The listing builds one solid part. Answer for the finished solid, in the listing's coordinates (mm). Face numbers are marked on the shaded views. Coordinates: 2 decimals unless noted, no trailing zeros. Loops run counter-clockwise (first coordinate to the right, second up) from the corner with the lowest first, then second, coordinate; pieces in that order, holes last. Notation, with made-up numbers: (64.25, 0.5) - (122.25, 0.5) arc R20 cw to (122.25, 35.5) - close; hole circle Ø5 at (42.25, 23.25). An arc over 180 degrees is marked (long way). One line per question, with ' | ' between items.
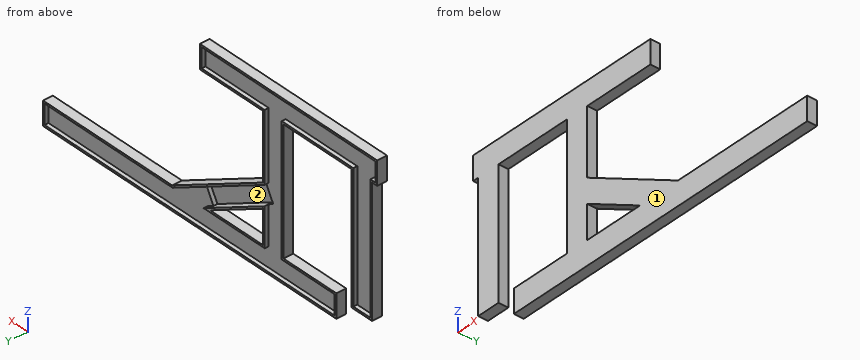
from build123d import *

# Parameters (mm, degrees)
SKETCH_3_W           = 10
SKETCH_3_H           = 65
SKETCH_3_W_2         = 85
SKETCH_3_H_2         = 10
EXTRUDE_2_DEPTH      = 1
EXTRUDE_3_DEPTH      = 4
EXTRUDE_3_DEPTH_BACK = 1
EXTRUDE_4_DEPTH      = 2
SKETCH_7_W           = 10
SKETCH_7_H           = 12
CUT_EXTRUDE_1_DEPTH  = 5
SKETCH_8_W           = 1
SKETCH_8_H           = 10
EXTRUDE_5_DEPTH      = 2
SKETCH_9_W           = 10
SKETCH_9_H           = 12
EXTRUDE_7_DEPTH      = 5
SKETCH_10_W          = 10
SKETCH_10_H          = 10
CUT_EXTRUDE_2_DEPTH  = 2


with BuildPart() as part:
    # 草图3 → 凸台-拉伸2 (new body)
    with BuildSketch(Plane(origin=(0, 0, 0), x_dir=(1, 0, 0), z_dir=(0, 1, 0))):
        with Locations((-68.5, -37.5)):
            Rectangle(SKETCH_3_W, SKETCH_3_H)
        Polygon((25.5, -70), (-11.5, -70), (-21.5, -70), (-63.5, -70), (-73.5, -70), (-76.5, -70), (-76.5, -80), (25.5, -80), align=None)
        Polygon((-11.5, -70), (-11.5, -34.745762712), (-16.5, -37.5), (-16.5, -27.5), (-11.5, -24.745762712), (-11.5, -5), (-21.5, -5), (-21.5, -70), align=None)
        Polygon((24.346153846, -5), (42.5, 5), (-42.5, 5), (-42.5, -5), (-21.5, -5), (-11.5, -5), align=None)
        with Locations((85, 0)):
            Rectangle(SKETCH_3_W_2, SKETCH_3_H_2)
        Polygon((24.346153846, -5), (42.5, -5), (42.5, 5), align=None)
        Polygon((-11.5, -34.745762712), (42.5, -5), (24.346153846, -5), (-11.5, -24.745762712), align=None)
        Polygon((-16.5, -37.5), (-11.5, -34.745762712), (-11.5, -24.745762712), (-16.5, -27.5), align=None)
    extrude(amount=EXTRUDE_2_DEPTH)

    # 草图4 → 凸台-拉伸3 (add, two sides)
    with BuildSketch(Plane(origin=(0, 1, 0), x_dir=(1, 0, 0), z_dir=(0, 1, 0))) as extrude_3_sk:
        Polygon((26.5, -69), (-10.5, -69), (-10.5, -35.336595122), (42.757203453, -6), (128.5, -6), (128.5, 6), (-43.5, 6), (-43.5, -6), (-22.5, -6), (-22.5, -69), (-62.5, -69), (-62.5, -4), (-74.5, -4), (-74.5, -69), (-77.5, -69), (-77.5, -81), (26.5, -81), align=None)
        Polygon((-11.5, -34.745762712), (42.5, -5), (127.5, -5), (127.5, 5), (-42.5, 5), (-42.5, -5), (-21.5, -5), (-21.5, -70), (-63.5, -70), (-63.5, -5), (-73.5, -5), (-73.5, -70), (-76.5, -70), (-76.5, -80), (25.5, -80), (25.5, -70), (-11.5, -70), align=None, mode=Mode.SUBTRACT)
        Polygon((-11.5, -5), (24.346153846, -5), (-11.5, -24.745762712), align=None)
        Polygon((-10.5, -23.053235386), (20.458181162, -6), (-10.5, -6), align=None, mode=Mode.SUBTRACT)
    extrude(amount=EXTRUDE_3_DEPTH)
    extrude(extrude_3_sk.sketch, amount=-EXTRUDE_3_DEPTH_BACK)

    # 草图5 → 凸台-拉伸4 (add)
    with BuildSketch(Plane(origin=(0, 1, 0), x_dir=(1, 0, 0), z_dir=(0, 1, 0))):
        Polygon((-10.007424518, -33.923581302), (-14.233552679, -26.251533255), (-11.5, -24.745762712), (-11.5, -5), (24.346153846, -5), (20.802538534, -6.951991486), (25.028666695, -14.624039532), (42.5, -5), (127.5, -5), (127.5, 5), (-42.5, 5), (-42.5, -5), (-21.5, -5), (-21.5, -70), (-63.5, -70), (-63.5, -5), (-73.5, -5), (-73.5, -70), (-76.5, -70), (-76.5, -80), (25.5, -80), (25.5, -70), (-11.5, -70), (-11.5, -34.745762712), align=None)
    extrude(amount=EXTRUDE_4_DEPTH)

    # 草图7 → 切除-拉伸1 (cut)
    with BuildSketch(Plane(origin=(0, 5, 0), x_dir=(1, 0, 0), z_dir=(0, 1, 0))):
        with Locations((123.5, 0)):
            Rectangle(SKETCH_7_W, SKETCH_7_H)
    extrude(amount=-CUT_EXTRUDE_1_DEPTH, mode=Mode.SUBTRACT)

    # 草图8 → 凸台-拉伸5 (add)
    with BuildSketch(Plane(origin=(0, 3, 0), x_dir=(1, 0, 0), z_dir=(0, 1, 0))):
        with Locations((118, 0)):
            Rectangle(SKETCH_8_W, SKETCH_8_H)
    extrude(amount=EXTRUDE_5_DEPTH)

    # 草图9 → 凸台-拉伸7 (add)
    with BuildSketch(Plane(origin=(0, 5, 0), x_dir=(1, 0, 0), z_dir=(0, 1, 0))):
        with Locations((-48.5, 0)):
            Rectangle(SKETCH_9_W, SKETCH_9_H)
    extrude(amount=-EXTRUDE_7_DEPTH)

    # 草图10 → 切除-拉伸2 (cut)
    with BuildSketch(Plane(origin=(0, 5, 0), x_dir=(1, 0, 0), z_dir=(0, 1, 0))):
        with Locations((-47.5, 0)):
            Rectangle(SKETCH_10_W, SKETCH_10_H)
    extrude(amount=-CUT_EXTRUDE_2_DEPTH, mode=Mode.SUBTRACT)


solid = part.part
Item 1: Find the intervals of material crossed by line 1 (X direction, y = 4.6, z = 66.5); line 2 (Z direction, x = -30, y = 4.4); line 3 (Z direction, x = 45.5, y = 3.1), in increasing order. Write a range as [from, to].
Taken from the geometry:
line 1: x = [-74.5, -73.5], [-63.5, -62.5], [-22.5, -21.5], [-11.5, -10.5] | line 2: z = [-6, -5], [5, 6], [69, 70], [80, 81] | line 3: z = [-6, -5], [5, 6]
Item 2: Find section C-C, the plane y = 3.9. State how many separate pieces and enclosed holes the cut face has, plus the area to 3 significant figures.
Taken from the geometry:
separate pieces: 2 | enclosed holes: 2 | area: 896 mm2
Item 3: Find section B-B, the plane x = -42. Write down the section's boundary in (y, z).
Taken from the geometry:
outline: (0, -6) - (5, -6) - (5, -5) - (3, -5) - (3, 5) - (5, 5) - (5, 6) - (0, 6) - close; (0, 69) - (5, 69) - (5, 70) - (3, 70) - (3, 80) - (5, 80) - (5, 81) - (0, 81) - close
Item 4: Find section A-A, the plane z = 29.5. Write down the section's boundary in (x, y).
Taken from the geometry:
outline: (-74.5, 0) - (-62.5, 0) - (-62.5, 5) - (-63.5, 5) - (-63.5, 3) - (-73.5, 3) - (-73.5, 5) - (-74.5, 5) - close; (-22.5, 0) - (0.1, 0) - (0.1, 5) - (-1.98, 5) - (-1.98, 1) - (-12.44, 1) - (-12.44, 3) - (-21.5, 3) - (-21.5, 5) - (-22.5, 5) - close
Item 5: Each of these flat-tipped pins is pushed along its axis until it touches: pin 1 Ø2 at (y, z) = (4, 50.5) entering from -X; pin 2 Ø2 at (y, z) = (3.5, 28.5) entering from +X; pin 3 Ø2 at (y, z) = (2, 44.5) entering from +X. Where does it stop, or does it pass through?
Taken from the geometry:
pin 1: stops at x = -74.5 | pin 2: stops at x = 3.73 | pin 3: stops at x = -10.5
Item 6: Find section D-D, the plane x = 62. Write down the section's boundary in (y, z), plus the area to 3 significant figures.
Taken from the geometry:
outline: (0, -6) - (5, -6) - (5, -5) - (3, -5) - (3, 5) - (5, 5) - (5, 6) - (0, 6) - close | area: 40.0 mm2
Item 7: The mould has two halves that part along Z. Classify the marked faces 1 and 2: pulls with the +Z half, pulls with the -Z half, needs draft (parallel to the pull), parting line crosses it, or undercut.
Taken from the geometry:
face 1: needs draft | face 2: undercut
